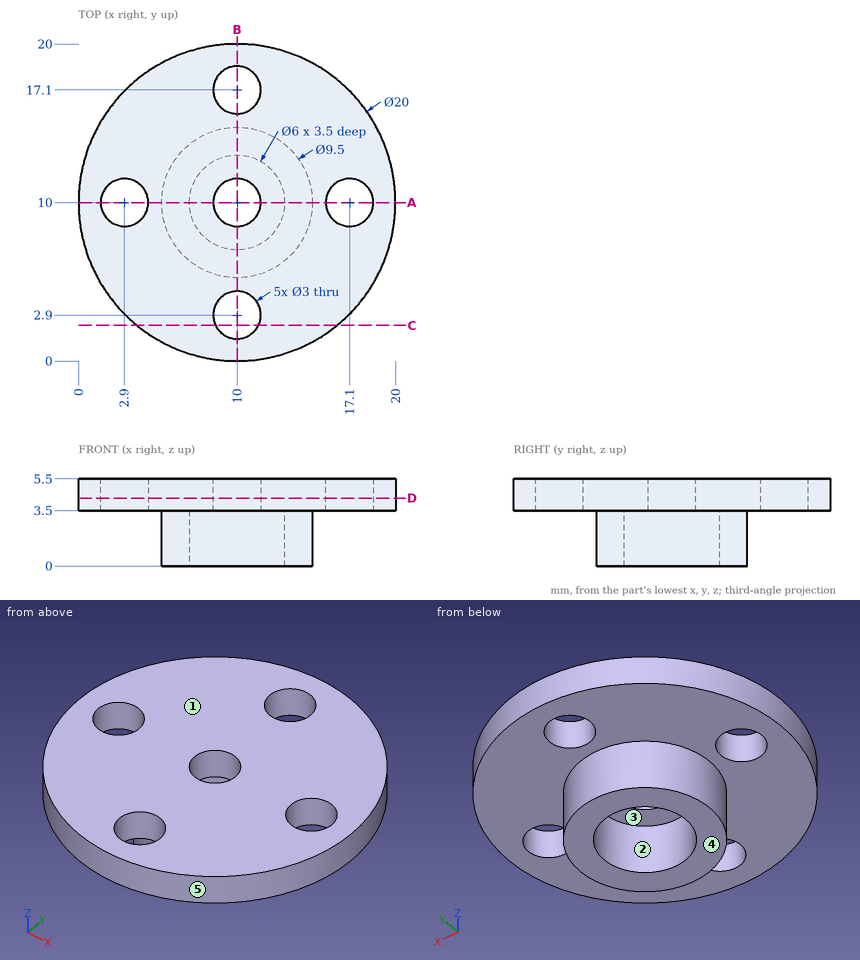
Answer from the drawing. Dimensions are ordinates in mm from the lowest x, y and z of the part. A direction names the side the tool comes from. Round coordinates to 2 decimals unless told otherwise and drop trailing zeros. Write each loop counter-clockwise with the first axis right and the second up, starting at its lowest first coordinate (ties: lowest second). Pieces come first, ordered by that corner, then holes. Notation, with made-up numbers: (24.25, 58) - (65.25, 58) arc R8 cw to (65.25, 66) - close; hole circle Ø8 at (18.5, 45). An arc over 180 degrees is marked (long way). Use a Markdown table: item, result.
(1) The part is cut by section A-A (y = 10). Write down the section's boundary in (x, z).
Reported:
| item | result |
|---|---|
| outline | (0, 3.5) - (1.4, 3.5) - (1.4, 5.5) - (0, 5.5) - close; (4.4, 3.5) - (5.25, 3.5) - (5.25, 0) - (7, 0) - (7, 3.5) - (8.5, 3.5) - (8.5, 5.5) - (4.4, 5.5) - close; (11.5, 3.5) - (13, 3.5) - (13, 0) - (14.75, 0) - (14.75, 3.5) - (15.6, 3.5) - (15.6, 5.5) - (11.5, 5.5) - close; (18.6, 3.5) - (20, 3.5) - (20, 5.5) - (18.6, 5.5) - close |
(2) This flat-tipped pin is pushed along its axis until it touches: pin 1 Ø3 at (x, y) = (9.5, 10) entering from -Z. Where does it stop, or does it pass through?
Reported:
| item | result |
|---|---|
| pin 1 | z = 3.5 |
(3) The part is cut by section C-C (y = 2.25). Write down the section's boundary in (x, z).
Reported:
| item | result |
|---|---|
| outline | (3.68, 3.5) - (8.65, 3.5) - (8.65, 5.5) - (3.68, 5.5) - close; (11.35, 3.5) - (16.32, 3.5) - (16.32, 5.5) - (11.35, 5.5) - close |
(4) Straight lines are drawn through the part: line 1 along Y through (x, z) = (10, 4.65); line 2 along Y through (x, z) = (10, 1.35); line 3 along Z through (x, y) = (3, 14). For each, find the intervals that lie inside material, in ascending order. Write a range as [from, to].
Reported:
| item | result |
|---|---|
| line 1 | [0, 1.4], [4.4, 8.5], [11.5, 15.6], [18.6, 20] |
| line 2 | [5.25, 7], [13, 14.75] |
| line 3 | [3.5, 5.5] |
(5) The part is cut by section D-D (z = 4.3). Write down the section's boundary in (x, y).
Reported:
| item | result |
|---|---|
| outline | circle Ø20 at (10, 10); hole circle Ø3 at (2.9, 10); hole circle Ø3 at (10, 2.9); hole circle Ø3 at (10, 10); hole circle Ø3 at (10, 17.1); hole circle Ø3 at (17.1, 10) |
(6) The mould has two halves that part along X. Classify the marked faces 3, 4 and 5: released by +X, released by -X, zero draft, split by the parting line, or undercut.
Reported:
| item | result |
|---|---|
| face 3 | undercut |
| face 4 | zero draft |
| face 5 | split by the parting line |
(7) Which of the six approach directions +Z, -Z, +X, -X, +Y, -Y give full straight-line access (tool end or side, diameter ignored) to the marked faces 1 and 2?
Reported:
| item | result |
|---|---|
| face 1 | +Z, +X, -X, +Y, -Y |
| face 2 | -Z |
